```python
from build123d import *

# Parameters (mm, degrees)
M4X0_7_TAPPED_HOLE1_D     = 3.3
M4X0_7_TAPPED_HOLE1_DEPTH = 10.1
M4X0_7_TAPPED_HOLE1_TIP   = 0.991420021
M4X0_7_TAPPED_HOLE2_D     = 3.3
M4X0_7_TAPPED_HOLE2_DEPTH = 10.1
M4X0_7_TAPPED_HOLE2_TIP   = 0.991420021


with BuildPart() as part:
    # Sketch1 → Revolve1 (revolve)
    with BuildSketch(Plane.XY, mode=Mode.PRIVATE) as revolve1_sk:
        Polygon((0, 12.7), (-15, 12.7), (-15, 0), (-30, 0), (-30, -12.7), (0, -12.7), align=None)
    revolve(revolve1_sk.sketch.rotate(Axis((0, -12.7, 0), (0, 1, 0)), 270), axis=Axis((0, -12.7, 0), (0, 1, 0)))

    # M4x0.7 Tapped Hole1
    with Locations(Plane(origin=(0, 12.7, 0), x_dir=(1, 0, 0), z_dir=(0, 1, 0))):
        with Locations((-10, 0), (5, 8.660254038), (5, -8.660254038)):
            Hole(M4X0_7_TAPPED_HOLE1_D / 2, depth=M4X0_7_TAPPED_HOLE1_DEPTH)
            with Locations((0, 0, -(M4X0_7_TAPPED_HOLE1_DEPTH + M4X0_7_TAPPED_HOLE1_TIP / 2))):  # 118° drill point
                Cone(0, M4X0_7_TAPPED_HOLE1_D / 2, M4X0_7_TAPPED_HOLE1_TIP, mode=Mode.SUBTRACT)

    # M4x0.7 Tapped Hole2
    with Locations(Plane(origin=(0, -12.7, 0), x_dir=(-1, 0, 0), z_dir=(0, -1, 0))):
        with Locations((-20, 0), (10, -17.320508076), (10, 17.320508076)):
            Hole(M4X0_7_TAPPED_HOLE2_D / 2, depth=M4X0_7_TAPPED_HOLE2_DEPTH)
            with Locations((0, 0, -(M4X0_7_TAPPED_HOLE2_DEPTH + M4X0_7_TAPPED_HOLE2_TIP / 2))):  # 118° drill point
                Cone(0, M4X0_7_TAPPED_HOLE2_D / 2, M4X0_7_TAPPED_HOLE2_TIP, mode=Mode.SUBTRACT)


solid = part.part
```
The model under review builds one solid part; all positions refer to its coordinate system, in mm. A direction names the side the tool comes from. Give positions to 0.01 mm unless a question says otherwise; leave off trailing zeros. Write each loop counter-clockwise with the first axis right and the second up, starting at its lowest first coordinate (ties: lowest second). Pieces come first, ordered by that corner, then holes. Notation, with made-up numbers: M -12,-38 L 43,-38 A18 ccw 43,-18 Z; hole C -20,20 d1. An arc over 180 degrees is marked long. Answer in a Markdown table with one row per item.
Item 1: Tool access review of faces 5 (the face through (0, -12.7, 0)), 6 (the face through (-10.36, -7.58, -15.71)), 7 (the face through (6.216, 7.579, -9.775)): name each direction out of +Z, -Z, +X, -X, +Y, -Y from which nothing blocks a thin tool from reaching the whole face with its end or side.
Check sheet entries:
| item | result |
|---|---|
| face 5 | +Z, -Z, +X, -X, -Y |
| face 6 | -Y |
| face 7 | +Y |
Item 2: Draft analysis for pull direction X (two halves, no side actions). For faces 1 (the face through (0, 12.7, 0)), 2 (the face through (5.15, 1.78, -8.9)), 3 (the face through (-11.524, 7.579, 0.632)), 4 (the face through (-1.32, -6.44, 29.97)), state which applies: +X half, -X half, draft (parallel to the pull), parting line (faces both ways), or undercut.
Check sheet entries:
| item | result |
|---|---|
| face 1 | draft |
| face 2 | undercut |
| face 3 | undercut |
| face 4 | parting line |
Item 3: Add section D-D on y = 10.25. Give the boundary of the cut face in (x, z), plus the area to 3 significant figures.
Check sheet entries:
| item | result |
|---|---|
| outline | C 0,0 d30; hole C -10,0 d3.3; hole C 5,-8.66 d3.3; hole C 5,8.66 d3.3 |
| area | 681 mm2 |
Item 4: For P1, Ø1.5, axis at y = 9.5, z = -7, coming from the +X side; P2, Ø1, axis at y = 8, z = 13, coming from the -X side; P3, Ø2, axis at x = 8.5, y = 8.5, coming from the -Z side; P4, Ø5, axis at x = -10, z = 11.5, coming from the +Y side, all flat-tipped, find the tip position at first contact; note any pin that passes through.
Check sheet entries:
| item | result |
|---|---|
| P1 | x = 13.64 |
| P2 | x = -8.29 |
| P3 | z = -12.99 |
| P4 | y = 12.7 |
Item 5: Add section B-B on y = -4.75. Give the boundary of the cut face in (x, z), plus the area to 3 significant figures.
Check sheet entries:
| item | result |
|---|---|
| outline | C 0,0 d60; hole C -10,-17.32 d3.3; hole C -10,17.32 d3.3; hole C 20,0 d3.3 |
| area | 2,800 mm2 |
Item 6: Add section C-C on x = 10.5. Give the boundary of the cut face in (y, z), plus the area to 3 significant figures.
Check sheet entries:
| item | result |
|---|---|
| outline | M -12.7,-28.1 L 0,-28.1 L 0,-10.71 L 12.7,-10.71 L 12.7,10.71 L 0,10.71 L 0,28.1 L -12.7,28.1 Z |
| area | 986 mm2 |
Item 7: Add section A-A on x = 0. Give the boundary of the cut face in (y, z).
Check sheet entries:
| item | result |
|---|---|
| outline | M -12.7,-30 L 0,-30 L 0,-15 L 12.7,-15 L 12.7,15 L 0,15 L 0,30 L -12.7,30 Z |
Item 8: For line 1 along Z through (x, y) = (5, 9); line 2 along Y through (x, z) = (-15, -12); line 3 along Z through (x, y) = (-10, 9.5), list the stretches that pass through material, from the lowest coordinate up.
Check sheet entries:
| item | result |
|---|---|
| line 1 | -14.14 to -10.31, -7.01 to 7.01, 10.31 to 14.14 |
| line 2 | -12.7 to 0 |
| line 3 | -11.18 to -1.65, 1.65 to 11.18 |
